Autodesk Inventor part; units mm, degrees
ref_plane "YZ Plane" through (0, 0, 0) normal (1, 0, 0) x (0, 1, 0)
ref_plane "XZ Plane" through (0, 0, 0) normal (0, 1, 0) x (-1, 0, 0)
ref_plane "XY Plane" through (0, 0, 0) normal (0, 0, 1) x (1, 0, 0)
sketch "Sketch1" plane through (0, 0, 0) normal (0, 1, 0) x (-1, 0, 0)
  line L0 (0, 0) -> (121.76, 0)
  line L1 (121.76, 0) -> (121.76, -220)
  line L2 (121.76, -220) -> (0, -220)
  line L3 (0, -220) -> (0, 0)
  line L4 (124.76, -223) -> (124.76, 3)
  line L5 (124.76, 3) -> (-3, 3)
  line L6 (-3, 3) -> (-3, -223)
  line L7 (-3, -223) -> (124.76, -223)
  circle A0 centre (5.08, -10.08) radius 1.6
  circle A1 centre (5.08, -10.08) radius 2.6
  circle A2 centre (55.88, -80.565) radius 2.5
  circle A3 centre (5.08, -151.05) radius 1.6
  circle A4 centre (5.08, -151.05) radius 2.6
  circle A5 centre (106.68, -10.08) radius 1.6
  circle A6 centre (106.68, -10.08) radius 2.6
  circle A7 centre (106.68, -151.05) radius 1.6
  circle A8 centre (106.68, -151.05) radius 2.6
  dimension "d0" = 121.76
  dimension "d1" = 220
  dimension "d2" = 3
  dimension "d22" = 3.2
  dimension "d23" = 1
  dimension "d24" = 5.08
  dimension "d25" = 10.08
  dimension "d26" = 5
  dimension "d35" = 3.2
  dimension "d36" = 1
  dimension "d37" = 140.97
  dimension "d38" = 0
  dimension "d39" = 3.2
  dimension "d40" = 1
  dimension "d41" = 101.6
  dimension "d42" = 0
  dimension "d43" = 3.2
  dimension "d44" = 1
  dimension "d45" = 0
  dimension "d46" = 0
  dimension "d47" = 50.8
  dimension "d48" = 70.485
extrude "Extrusion1" add sketch "Sketch1" along normal blind 15 contours L0 L1 L2 L3 | A0 | A1 | A2 | A3 | A4 | A5 | A6 | A7 | A8
extrude "Extrusion2" add sketch "Sketch1" along normal blind 40 contours L7 L6 L5 L4
fillet "Fillet1" radius 3 4 edges at (3, 20, -223) (-124.76, 20, -223) (-124.76, 20, 3) (3, 20, 3)
sketch "Sketch2" plane through (3, 0, 0) normal (1, 0, 0) x (0, 0, -1)
  line L0 (220, 15) -> (0, 15) construction
  line L1 (0, 15) -> (220, 15)
  line L2 (73.9, 33.95) -> (86, 33.95)
  line L3 (86, 33.95) -> (86, 23.2)
  line L4 (86, 23.2) -> (73.9, 23.2)
  line L5 (73.9, 23.2) -> (73.9, 33.95)
  line L6 (106.15, 33.95) -> (114.9, 33.95)
  line L7 (114.9, 33.95) -> (114.9, 23.2)
  line L8 (114.9, 23.2) -> (106.15, 23.2)
  line L9 (106.15, 23.2) -> (106.15, 33.95)
  line L10 (0, 0) -> (0, 40)
  line L11 (30.85, 25.9) -> (38.15, 25.9)
  line L12 (38.15, 25.9) -> (38.15, 23.1)
  line L13 (38.15, 23.1) -> (30.85, 23.1)
  line L14 (30.85, 23.1) -> (30.85, 25.9)
  line L15 (110, 15) -> (110, 0) construction
  line L16 (220, 0) -> (0, 0)
  line L17 (48.413, 0) -> (43.7499, 10)
  line L18 (43.7499, 10) -> (66.2501, 10)
  line L19 (66.2501, 10) -> (61.587, 0)
  line L20 (48.413, 0) -> (61.587, 0)
  line L21 (55, 0) -> (55, 15) construction
  line L22 (171.587, 0) -> (176.2501, 10)
  line L23 (176.2501, 10) -> (153.7499, 10)
  line L24 (153.7499, 10) -> (158.413, 0)
  line L25 (171.587, 0) -> (158.413, 0)
  point P0 (110, 7.5)
  point P1 (55, 0)
  point P2 (158.413, 0)
  dimension "d9" = 12.1
  dimension "d10" = 10.75
  dimension "d11" = 8.2
  dimension "d12" = 8.75
  dimension "d13" = 10.75
  dimension "d14" = 8.2
  dimension "d15" = 20.15
  dimension "d19" = 7.3
  dimension "d20" = 2.8
  dimension "d21" = 8.1
  dimension "d49" = 35.75
  dimension "d50" = 30.85
  dimension "d72" = 13.174
  dimension "d73" = 65
  dimension "d74" = 65
  dimension "d75" = 10
  dimension "d76" = 55
extrude "Extrusion3" cut sketch "Sketch2" against normal up to surface (3 mm away) contours L2 L3 L4 L5 | L6 L7 L8 L9 | L11 L12 L13 L14
extrude "Extrusion4" add sketch "Sketch1" along normal blind 20 contours A1 | A2 | A4 | A6 | A8
sketch "Sketch3" plane through (0, 40, 0) normal (0, 1, 0) x (1, 0, 0)
  line L0 (-121.76, 0) -> (-121.76, 220)
  line L1 (-121.76, 110) -> (0, 110) construction
  line L2 (0, 220) -> (0, 0)
  line L3 (-121.76, 0) -> (0, 0)
  line L4 (-60.88, 0) -> (-60.88, 220) construction
  line L5 (-121.76, 220) -> (0, 220)
  line L6 (0, 0) -> (-10, 0)
  line L7 (-10, 0) -> (-10, 10)
  line L8 (-10, 10) -> (0, 10)
  line L9 (0, 10) -> (0, 0)
  line L10 (-121.76, 0) -> (-111.76, 0)
  line L11 (-111.76, 0) -> (-111.76, 10)
  line L12 (-111.76, 10) -> (-121.76, 10)
  line L13 (-121.76, 10) -> (-121.76, 0)
  line L14 (0, 220) -> (-10, 220)
  line L15 (-10, 220) -> (-10, 210)
  line L16 (-10, 210) -> (0, 210)
  line L17 (0, 210) -> (0, 220)
  line L18 (-121.76, 220) -> (-111.76, 220)
  line L19 (-111.76, 220) -> (-111.76, 210)
  line L20 (-111.76, 210) -> (-121.76, 210)
  line L21 (-121.76, 210) -> (-121.76, 220)
  line L22 (-121.76, 0) -> (0, 0)
  line L23 (0, 0) -> (0, 220)
  line L24 (0, 220) -> (-121.76, 220)
  line L25 (-121.76, 220) -> (-121.76, 0)
  point P0 (0, 210)
  dimension "d51" = 10
  dimension "d52" = 10
extrude "Extrusion6" add sketch "Sketch3" against normal blind 10 contours L0 L12 L11 L3 | L0 L5 L19 L20 | L7 L8 L2 L3 | L5 L2 L16 L15
sketch "Sketch4" plane through (0, 40, 0) normal (0, 1, 0) x (1, 0, 0)
  line L0 (-10, 10) -> (-10, 0)
  line L1 (0, 10) -> (-10, 10)
  line L2 (-10, 220) -> (-10, 210)
  line L3 (-10, 210) -> (0, 210)
  line L4 (-121.76, 210) -> (-111.76, 210)
  line L5 (-111.76, 210) -> (-111.76, 220)
  line L6 (-111.76, 0) -> (-111.76, 10)
  line L7 (-111.76, 10) -> (-121.76, 10)
  point P0 (0, 0)
  point P1 (-5, 5)
  point P2 (-116.76, 5)
  point P3 (-116.76, 215)
  point P4 (-5, 215)
  dimension "d55" = 5
  dimension "d63" = 5
  dimension "d64" = 5
  dimension "d65" = 5
  dimension "d66" = 5
  dimension "d67" = 5
  dimension "d68" = 5
  dimension "d69" = 5
hole "Hole1" at (-5, 40, -5) at (-5, 40, -215) at (-116.76, 40, -215) at (-116.76, 40, -5) direction (0, -1, 0) diameter 3 depth 10
extrude "Extrusion7" cut sketch "Sketch3" against normal blind 3
extrude "Extrusion8" cut sketch "Sketch2" against normal up to surface (127.76 mm away) contours L16 L17 L18 L19 | L16 L24 L23 L22
extrude "Extrusion9" add sketch "Sketch2" against normal blind 2.5 contours L16 L17 L18 L19 | L16 L24 L23 L22
sketch "Sketch5" plane through (-121.76, 0, 3) normal (0, 0, 1) x (1, 0, 0)
  line L0 (122.26, 10) -> (-3, 10)
  line L1 (59.63, 10) -> (59.63, 0) construction
  line L2 (-3, 0) -> (122.26, 0)
  line L3 (29.815, 10) -> (29.815, 0) construction
  line L4 (23.228, 0) -> (36.402, 0)
  line L5 (36.402, 0) -> (41.0651, 10)
  line L6 (41.0651, 10) -> (18.5649, 10)
  line L7 (18.5649, 10) -> (23.228, 0)
  line L8 (89.445, 10) -> (89.445, 0) construction
  line L9 (96.032, 0) -> (82.858, 0)
  line L10 (82.858, 0) -> (78.1949, 10)
  line L11 (78.1949, 10) -> (100.6951, 10)
  line L12 (100.6951, 10) -> (96.032, 0)
  point P0 (121.76, 0)
  point P1 (59.63, 5)
  point P2 (18.5649, 10)
  point P3 (41.0651, 10)
  dimension "d81" = 29.815
  dimension "d82" = 13.174
  dimension "d83" = 65
  dimension "d84" = 65
  dimension "d85" = 10
extrude "Extrusion10" cut sketch "Sketch5" against normal up to surface (226 mm away) contours L12 L2 L10 L0 | L5 L2 L7 L0
extrude "Extrusion11" add sketch "Sketch5" against normal blind 2.5 contours L12 L2 L10 L0 | L5 L2 L7 L0
properties part number "Base"
Geometry: final body of the model. Coordinates: model frame, mm. A direction names the side the tool comes from. Coordinates: 2 decimals unless noted, no trailing zeros. Order: outer loops, then holes, each group sorted by start corner. A loop starts at its lowest first (then second) coordinate and runs counter-clockwise, first axis right, second up. Notation, with made-up numbers: (80.25, 59) - (130.25, 59) arc R6 ccw to (130.25, 63) - close; hole circle Ø6 at (-4.5, 38.25). An arc over 180 degrees is marked (long way). Write each question's results on one line, items separated by ' | '.
1) Pin query (flat end, axial travel): pin 1 (5.5 mm diameter, centred on x = -5, z = -151, fed in from +Y); pin 2 (8 mm diameter, centred on x = -88.5, y = 4.5, fed in from -Z); pin 3 (5 mm diameter, centred on x = -101.5, z = -97.5, fed in from +Y). Return the tip coordinate at first contact, or that it passes through.
Results list:
pin 1: y = 20 | pin 2: z = 0.5 | pin 3: y = 15
2) Section A-A, the plane x = -55.88. Return loops of the section in (y, z) (3 decimals).
Results list:
outline: (0, -223) - (40, -223) - (40, -220) - (15, -220) - (15, -83.065) - (20, -83.065) - (20, -78.065) - (15, -78.065) - (15, 0) - (40, 0) - (40, 3) - (0, 3) - (0, -48.413) - (10, -43.75) - (10, -66.25) - (0, -61.587) - (0, -158.413) - (10, -153.75) - (10, -176.25) - (0, -171.587) - close
3) Set-up query: faces 4 (the flat face through (-100.896, 5.07, -196.934)), 5 (the flat face through (-111.46, 5.07, -156.05)), 6 (the flat face through (-10, 34, -215)), 7 (the flat face through (-6.2, 30, -216.2)). Return all of +Z, -Z, +X, -X, +Y, -Y with unobstructed straight access to the full face (end or side cutting, diameter ignored); none if empty.
Results list:
face 4: -Z | face 5: -X | face 6: +Y | face 7: none
4) Section C-C, the plane x = -14. Return loops of the section in (y, z), plus the area to 3 significant figures.
Results list:
outline: (0, -223) - (40, -223) - (40, -220) - (15, -220) - (15, 0) - (40, 0) - (40, 3) - (0, 3) - (0, -48.41) - (10, -43.75) - (10, -66.25) - (0, -61.59) - (0, -158.41) - (10, -153.75) - (10, -176.25) - (0, -171.59) - close | area: 3,180 mm^2
5) Pull-direction query (Z, two-part tool) for faces 1 (the flat face through (-12.43, 5.07, -63.95)), 2 (the flat face through (3, 20, -108)), 3 (the flat face through (-62, 20, 3)); classes: pulls with the +Z half, pulls with the -Z half, needs draft (parallel to the pull), parting line crosses it, or undercut.
Results list:
face 1: undercut | face 2: needs draft | face 3: pulls with the +Z half
6) Section B-B, the plane z = -194. Return loops of the section in (x, y).
Results list:
outline: (-124.76, 0) - (-98.53, 0) - (-103.2, 10) - (-80.69, 10) - (-85.36, 0) - (-38.9, 0) - (-43.57, 10) - (-21.06, 10) - (-25.73, 0) - (3, 0) - (3, 40) - (0, 40) - (0, 15) - (-121.76, 15) - (-121.76, 40) - (-124.76, 40) - close
7) Section D-D, the plane y = 4.5. State how many separate pieces and enclosed holes the cut face has, plus the area to 3 significant figures.
Results list:
separate pieces: 5 | enclosed holes: 0 | area: 18,000 mm^2
8) Line query: line 1 (Z direction, x = -5, y = 32); line 2 (X direction, y = 18.8, z = -151.05); line 3 (Z direction, x = -106.68, y = 17.95). Output: solid intervals per line, ascending. Write a range as from..to.
Results list:
line 1: -223..-216.5, -213.5..-210, -10..-6.5, -3.5..3 | line 2: -124.76..-121.76, -109.28..-108.28, -105.08..-104.08, -7.68..-6.68, -3.48..-2.48, 0..3 | line 3: -223..-220, -153.65..-152.65, -149.45..-148.45, -12.68..-11.68, -8.48..-7.48, 0..3
